from build123d import *

# Parameters (mm, degrees)
F0_W     = 1.27
F0_H     = 22.86
F1_DEPTH = 24.13
F0_H_2   = 11.43
F0_W_2   = 22.86
F0_H_3   = 1.27
F2_DEPTH = 25.4
F3_DEPTH = 3.81
F4_SCALE = 0.5


with BuildPart() as f1:
    # F0 (on Top) → F1 (new body)
    with BuildSketch(Plane.XY):
        with Locations((26.035, 12.7)):
            Rectangle(F0_W, F0_H)
    extrude(amount=F1_DEPTH)



with BuildPart() as f1b:
    # F0 (on Top) → F1, piece 2 (new body)
    with BuildSketch(Plane.XY):
        with Locations((52.705, 12.7)):
            Rectangle(F0_W, F0_H)
    extrude(amount=F1_DEPTH)


with BuildPart() as f1c:
    # F0 (on Top) → F1, piece 3 (new body)
    with BuildSketch(Plane.XY):
        with Locations((79.375, 12.7)):
            Rectangle(F0_W, F0_H)
    extrude(amount=F1_DEPTH)


with BuildPart() as f1d:
    # F0 (on Top) → F1, piece 4 (new body)
    with BuildSketch(Plane.XY):
        with Locations((106.045, 6.985)):
            Rectangle(F0_W, F0_H_2)
        with Locations((106.045, 18.415)):
            Rectangle(F0_W, F0_H_2)
    extrude(amount=F1_DEPTH)


with BuildPart() as f1e:
    # F0 (on Top) → F1, piece 5 (new body)
    with BuildSketch(Plane.XY):
        with Locations((119.38, 26.035)):
            Rectangle(F0_W_2, F0_H_3)
    extrude(amount=F1_DEPTH)


with BuildPart() as f1f:
    # F0 (on Top) → F1, piece 6 (new body)
    with BuildSketch(Plane.XY):
        with Locations((119.38, 52.705)):
            Rectangle(F0_W_2, F0_H_3)
    extrude(amount=F1_DEPTH)


with BuildPart() as f1g:
    # F0 (on Top) → F1, piece 7 (new body)
    with BuildSketch(Plane.XY):
        with Locations((119.38, 79.375)):
            Rectangle(F0_W_2, F0_H_3)
    extrude(amount=F1_DEPTH)


with BuildPart() as f1h:
    # F0 (on Top) → F1, piece 8 (new body)
    with BuildSketch(Plane.XY):
        with Locations((119.38, 106.045)):
            Rectangle(F0_W_2, F0_H_3)
    extrude(amount=F1_DEPTH)


with BuildPart() as f1i:
    # F0 (on Top) → F1, piece 9 (new body)
    with BuildSketch(Plane.XY):
        with Locations((132.715, 119.38)):
            Rectangle(F0_W, F0_H)
    extrude(amount=F1_DEPTH)


with BuildPart() as f1j:
    # F0 (on Top) → F1, piece 10 (new body)
    with BuildSketch(Plane.XY):
        with Locations((159.385, 119.38)):
            Rectangle(F0_W, F0_H)
    extrude(amount=F1_DEPTH)


with BuildPart() as f1k:
    # F0 (on Top) → F1, piece 11 (new body)
    with BuildSketch(Plane.XY):
        with Locations((186.055, 119.38)):
            Rectangle(F0_W, F0_H)
    extrude(amount=F1_DEPTH)


with BuildPart() as f1l:
    # F0 (on Top) → F1, piece 12 (new body)
    with BuildSketch(Plane.XY):
        with Locations((212.725, 119.38)):
            Rectangle(F0_W, F0_H)
    extrude(amount=F1_DEPTH)


with BuildPart() as f1m:
    # F0 (on Top) → F1, piece 13 (new body)
    with BuildSketch(Plane.XY):
        with Locations((239.395, 119.38)):
            Rectangle(F0_W, F0_H)
    extrude(amount=F1_DEPTH)


with BuildPart() as f1n:
    # F0 (on Top) → F1, piece 14 (new body)
    with BuildSketch(Plane.XY):
        with Locations((266.065, 119.38)):
            Rectangle(F0_W, F0_H)
    extrude(amount=F1_DEPTH)


with BuildPart() as f1o:
    # F0 (on Top) → F1, piece 15 (new body)
    with BuildSketch(Plane.XY):
        with Locations((292.735, 119.38)):
            Rectangle(F0_W, F0_H)
    extrude(amount=F1_DEPTH)


with BuildPart() as f1_1:
    add(f1.part)

    add(f1b.part)  # F2 merges F1b

    add(f1c.part)  # F2 merges F1c

    add(f1d.part)  # F2 merges F1d

    add(f1e.part)  # F2 merges F1e

    add(f1f.part)  # F2 merges F1f

    add(f1g.part)  # F2 merges F1g

    add(f1h.part)  # F2 merges F1h

    add(f1i.part)  # F2 merges F1i

    add(f1j.part)  # F2 merges F1j

    add(f1k.part)  # F2 merges F1k

    add(f1l.part)  # F2 merges F1l

    add(f1m.part)  # F2 merges F1m

    add(f1n.part)  # F2 merges F1n

    add(f1o.part)  # F2 merges F1o
    # F0 (on Top) → F2 (join)
    with BuildSketch(Plane.XY):
        Polygon((0, 25.4), (0, 0), (25.4, 0), (25.4, 1.27), (25.4, 24.13), (25.4, 25.4), align=None)
        Polygon((26.67, 24.13), (26.67, 1.27), (26.67, 0), (52.07, 0), (52.07, 1.27), (52.07, 24.13), (52.07, 25.4), (26.67, 25.4), align=None)
        Polygon((53.34, 24.13), (53.34, 1.27), (53.34, 0), (78.74, 0), (78.74, 1.27), (78.74, 24.13), (78.74, 25.4), (53.34, 25.4), align=None)
        Polygon((80.01, 24.13), (80.01, 1.27), (80.01, 0), (105.41, 0), (105.41, 1.27), (105.41, 12.7), (105.41, 24.13), (105.41, 25.4), (80.01, 25.4), align=None)
        Polygon((106.68, 12.7), (106.68, 1.27), (106.68, 0), (132.08, 0), (132.08, 25.4), (130.81, 25.4), (107.95, 25.4), (106.68, 25.4), (106.68, 24.13), align=None)
        Polygon((106.68, 26.67), (107.95, 26.67), (130.81, 26.67), (132.08, 26.67), (132.08, 52.07), (130.81, 52.07), (107.95, 52.07), (106.68, 52.07), align=None)
        Polygon((106.68, 53.34), (107.95, 53.34), (130.81, 53.34), (132.08, 53.34), (132.08, 78.74), (130.81, 78.74), (107.95, 78.74), (106.68, 78.74), align=None)
        Polygon((106.68, 80.01), (107.95, 80.01), (130.81, 80.01), (132.08, 80.01), (132.08, 105.41), (130.81, 105.41), (107.95, 105.41), (106.68, 105.41), align=None)
        Polygon((106.68, 106.68), (107.95, 106.68), (130.81, 106.68), (132.08, 106.68), (132.08, 107.95), (132.08, 130.81), (132.08, 132.08), (106.68, 132.08), align=None)
        Polygon((133.35, 130.81), (133.35, 107.95), (133.35, 106.68), (158.75, 106.68), (158.75, 107.95), (158.75, 130.81), (158.75, 132.08), (133.35, 132.08), align=None)
        Polygon((160.02, 130.81), (160.02, 107.95), (160.02, 106.68), (185.42, 106.68), (185.42, 107.95), (185.42, 130.81), (185.42, 132.08), (160.02, 132.08), align=None)
        Polygon((186.69, 130.81), (186.69, 107.95), (186.69, 106.68), (212.09, 106.68), (212.09, 107.95), (212.09, 130.81), (212.09, 132.08), (186.69, 132.08), align=None)
        Polygon((213.36, 130.81), (213.36, 107.95), (213.36, 106.68), (238.76, 106.68), (238.76, 107.95), (238.76, 130.81), (238.76, 132.08), (213.36, 132.08), align=None)
        Polygon((240.03, 130.81), (240.03, 107.95), (240.03, 106.68), (265.43, 106.68), (265.43, 107.95), (265.43, 130.81), (265.43, 132.08), (240.03, 132.08), align=None)
        Polygon((266.7, 130.81), (266.7, 107.95), (266.7, 106.68), (292.1, 106.68), (292.1, 107.95), (292.1, 130.81), (292.1, 132.08), (266.7, 132.08), align=None)
        Polygon((293.37, 130.81), (293.37, 107.95), (293.37, 106.68), (318.77, 106.68), (318.77, 107.95), (318.77, 130.81), (318.77, 132.08), (293.37, 132.08), align=None)
    extrude(amount=F2_DEPTH)

    # F0 (on Top) → F3 (join)
    with BuildSketch(Plane.XY):
        Polygon((53.34, 24.13), (53.34, 1.27), (53.34, 0), (78.74, 0), (78.74, 1.27), (78.74, 24.13), (78.74, 25.4), (53.34, 25.4), align=None)
        Polygon((213.36, 130.81), (213.36, 107.95), (213.36, 106.68), (238.76, 106.68), (238.76, 107.95), (238.76, 130.81), (238.76, 132.08), (213.36, 132.08), align=None)
        Polygon((106.68, 106.68), (107.95, 106.68), (130.81, 106.68), (132.08, 106.68), (132.08, 107.95), (132.08, 130.81), (132.08, 132.08), (106.68, 132.08), align=None)
        Polygon((0, 25.4), (0, 0), (25.4, 0), (25.4, 1.27), (25.4, 24.13), (25.4, 25.4), align=None)
        Polygon((293.37, 130.81), (293.37, 107.95), (293.37, 106.68), (318.77, 106.68), (318.77, 107.95), (318.77, 130.81), (318.77, 132.08), (293.37, 132.08), align=None)
        Polygon((106.68, 80.01), (107.95, 80.01), (130.81, 80.01), (132.08, 80.01), (132.08, 105.41), (130.81, 105.41), (107.95, 105.41), (106.68, 105.41), align=None)
        Polygon((106.68, 53.34), (107.95, 53.34), (130.81, 53.34), (132.08, 53.34), (132.08, 78.74), (130.81, 78.74), (107.95, 78.74), (106.68, 78.74), align=None)
        Polygon((106.68, 26.67), (107.95, 26.67), (130.81, 26.67), (132.08, 26.67), (132.08, 52.07), (130.81, 52.07), (107.95, 52.07), (106.68, 52.07), align=None)
        Polygon((26.67, 24.13), (26.67, 1.27), (26.67, 0), (52.07, 0), (52.07, 1.27), (52.07, 24.13), (52.07, 25.4), (26.67, 25.4), align=None)
        Polygon((160.02, 130.81), (160.02, 107.95), (160.02, 106.68), (185.42, 106.68), (185.42, 107.95), (185.42, 130.81), (185.42, 132.08), (160.02, 132.08), align=None)
        Polygon((186.69, 130.81), (186.69, 107.95), (186.69, 106.68), (212.09, 106.68), (212.09, 107.95), (212.09, 130.81), (212.09, 132.08), (186.69, 132.08), align=None)
        Polygon((240.03, 130.81), (240.03, 107.95), (240.03, 106.68), (265.43, 106.68), (265.43, 107.95), (265.43, 130.81), (265.43, 132.08), (240.03, 132.08), align=None)
        Polygon((106.68, 12.7), (106.68, 1.27), (106.68, 0), (132.08, 0), (132.08, 25.4), (130.81, 25.4), (107.95, 25.4), (106.68, 25.4), (106.68, 24.13), align=None)
        Polygon((133.35, 130.81), (133.35, 107.95), (133.35, 106.68), (158.75, 106.68), (158.75, 107.95), (158.75, 130.81), (158.75, 132.08), (133.35, 132.08), align=None)
        Polygon((80.01, 24.13), (80.01, 1.27), (80.01, 0), (105.41, 0), (105.41, 1.27), (105.41, 12.7), (105.41, 24.13), (105.41, 25.4), (80.01, 25.4), align=None)
        Polygon((266.7, 130.81), (266.7, 107.95), (266.7, 106.68), (292.1, 106.68), (292.1, 107.95), (292.1, 130.81), (292.1, 132.08), (266.7, 132.08), align=None)
        with Locations((132.715, 119.38)):
            Rectangle(F0_W, F0_H)
        with Locations((119.38, 106.045)):
            Rectangle(F0_W_2, F0_H_3)
        with Locations((239.395, 119.38)):
            Rectangle(F0_W, F0_H)
        with Locations((186.055, 119.38)):
            Rectangle(F0_W, F0_H)
        with Locations((159.385, 119.38)):
            Rectangle(F0_W, F0_H)
        with Locations((52.705, 12.7)):
            Rectangle(F0_W, F0_H)
        with Locations((212.725, 119.38)):
            Rectangle(F0_W, F0_H)
        with Locations((119.38, 79.375)):
            Rectangle(F0_W_2, F0_H_3)
        with Locations((119.38, 52.705)):
            Rectangle(F0_W_2, F0_H_3)
        with Locations((119.38, 26.035)):
            Rectangle(F0_W_2, F0_H_3)
        with Locations((79.375, 12.7)):
            Rectangle(F0_W, F0_H)
        with Locations((26.035, 12.7)):
            Rectangle(F0_W, F0_H)
        with Locations((266.065, 119.38)):
            Rectangle(F0_W, F0_H)
        with Locations((106.045, 6.985)):
            Rectangle(F0_W, F0_H_2)
        with Locations((292.735, 119.38)):
            Rectangle(F0_W, F0_H)
        with Locations((106.045, 18.415)):
            Rectangle(F0_W, F0_H_2)
    extrude(amount=-F3_DEPTH)


with BuildPart() as f1_2:
    # F4: moved
    add(f1_1.part.scale(F4_SCALE))


solid = f1_2.part
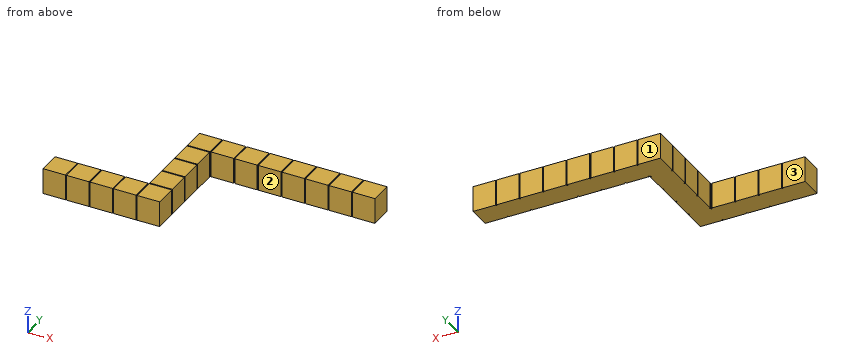
Read the model definition and answer for the solid it produces. Units are mm, in the model's axes. Face numbers are marked on the shaded views. A direction names the side the tool comes from. Coordinates: 2 decimals unless noted, no trailing zeros. Loops run counter-clockwise (first coordinate to the right, second up) from the corner with the lowest first, then second, coordinate; pieces in that order, holes last. Notation, with made-up numbers: (-12, 41.25) -> (-8, 41.25) arc R26 ccw to (-8, 59.25) -> close; hole circle Ø8 at (-11, 20). An arc over 180 degrees is marked (long way). Answer in a Markdown table with one row per item.
Item 1: Each of these flat-tipped pins is pushed along its axis until it touches: P1, Ø5, axis at y = 19, z = 4.5, coming from the -X side; P2, Ø0.7, axis at x = 66.5, z = 5.5, coming from the -Y side; P3, Ø2, axis at x = 112.5, y = 53, coming from the -Z side (3 decimals); P4, Ø4, axis at x = 19, z = 6, coming from the +Y side. Where does it stop, or does it pass through?
Returned:
| item | result |
|---|---|
| P1 | stops at x = 53.34 |
| P2 | stops at y = 53.34 |
| P3 | stops at z = -1.905 |
| P4 | stops at y = 12.7 |
Item 2: A cutting plane is placed at A-A on x = 129. Determine the outline of the cut face in (y, z) (3 decimals), plus the area to 3 significant figures.
Returned:
| item | result |
|---|---|
| outline | (53.34, -1.905) -> (66.04, -1.905) -> (66.04, 12.7) -> (53.34, 12.7) -> close |
| area | 185 mm^2 |
Item 3: Straight lines are drawn through the part: line 1 along X through (y, z) = (60, 7.75) (3 decimals); line 2 along Y through (x, z) = (11, 10); line 3 along X through (y, z) = (8.5, 3.5). For each, find the intervals that lie inside material, in ascending order. Write a range as [from, to].
Returned:
| item | result |
|---|---|
| line 1 | x = [53.34, 159.385] |
| line 2 | y = [0, 12.7] |
| line 3 | x = [0, 66.04] |
Item 4: For the marked faces 1, 2 and 3, determine the directions among +Z, -Z, +X, -X, +Y, -Y from which every point of the face is accessible in a straight line to the end or side of a thin tool.
Returned:
| item | result |
|---|---|
| face 1 | +Z, -Z, +X, -X, +Y |
| face 2 | +Z, -Z, +X, -Y |
| face 3 | +Z, -Z, -X, +Y |
